Geometry: final body of the model. Coordinates: model frame, mm. Coordinates: 2 decimals unless noted, no trailing zeros. Write each loop counter-clockwise with the first axis right and the second up, starting at its lowest first coordinate (ties: lowest second). Pieces come first, ordered by that corner, then holes. Notation, with made-up numbers: (59.25, 30.5) -> (74.25, 30.5) arc R27 cw to (74.25, 66.5) -> close; hole circle Ø6 at (-8, 82). An arc over 180 degrees is marked (long way). One line per item, written item: value. Start each with the question number.
from build123d import *

# Parameters (mm, degrees)
SKETCH_1_R          = 1.6
EXTRUDE_1_DEPTH     = 3
SKETCH_3_R          = 1.6
CUT_EXTRUDE_1_DEPTH = 92.290744328
FILLET_1_R          = 1
SKETCH_4_W          = 12
SKETCH_4_H          = 3
CUT_EXTRUDE_2_DEPTH = 92.290744328
SKETCH_5_R          = 1
CUT_EXTRUDE_3_DEPTH = 92.290744328
CUT_EXTRUDE_4_DEPTH = 92.290744328
SKETCH_7_R          = 1.6
SKETCH_7_W          = 3
SKETCH_7_H          = 9
EXTRUDE_2_DEPTH     = 3
FILLET_3_R          = 2
SKETCH_8_R          = 1
CUT_EXTRUDE_5_DEPTH = 130.100735862


with BuildPart() as part:
    # 草图1 → 凸台-拉伸1 (new body)
    with BuildSketch(Plane(origin=(0, 0, 0), x_dir=(1, 0, 0), z_dir=(0, 1, 0))):
        Polygon((-90, -15), (-72.5, -15), (-72.5, 0.5), (72.5, 0.5), (72.5, -15), (90, -15), (90, 15), (-90, 15), align=None)
        with Locations(Location((78, -10, 0), (0, 0, 270))):
            Circle(SKETCH_1_R, mode=Mode.SUBTRACT)
        with Locations(Location((-78, -10, 0), (0, 0, 90))):
            Circle(SKETCH_1_R, mode=Mode.SUBTRACT)
        with Locations(Location((-83, 10, 0), (0, 0, 270))):
            Circle(SKETCH_1_R, mode=Mode.SUBTRACT)
        with Locations(Location((83, 10, 0), (0, 0, 90))):
            Circle(SKETCH_1_R, mode=Mode.SUBTRACT)
    extrude(amount=EXTRUDE_1_DEPTH)

    # 草图3 → 切除-拉伸1 (cut, through all)
    with BuildSketch(Plane(origin=(0, 3, 0), x_dir=(1, 0, 0), z_dir=(0, 1, 0))):
        with Locations(Location((87, -4.5, 0), (0, 0, 90))):
            Circle(SKETCH_3_R)
        with Locations(Location((-87, -4.5, 0), (0, 0, 270))):
            Circle(SKETCH_3_R)
    extrude(amount=-CUT_EXTRUDE_1_DEPTH, mode=Mode.SUBTRACT)

    # 圆角1
    fillet_1_edges = [part.edges().sort_by_distance(p)[0] for p in [
        (72.5, 1.5, -0.5),
        (-72.5, 1.5, -0.5),
    ]]
    fillet(fillet_1_edges, radius=FILLET_1_R)

    # 草图4 → 切除-拉伸2 (cut, through all)
    with BuildSketch(Plane.XZ):
        with Locations((60, -7.5)):
            Rectangle(SKETCH_4_W, SKETCH_4_H)
        with Locations((30, -7.5)):
            Rectangle(SKETCH_4_W, SKETCH_4_H)
        with Locations((0, -7.5)):
            Rectangle(SKETCH_4_W, SKETCH_4_H)
        with Locations((-30, -7.5)):
            Rectangle(SKETCH_4_W, SKETCH_4_H)
        with Locations((-60, -7.5)):
            Rectangle(SKETCH_4_W, SKETCH_4_H)
    extrude(amount=-CUT_EXTRUDE_2_DEPTH, mode=Mode.SUBTRACT)

    # 草图5 → 切除-拉伸3 (cut, through all)
    with BuildSketch(Plane.XZ):
        with Locations((65, -9)):
            Circle(SKETCH_5_R)
        with Locations((55, -9)):
            Circle(SKETCH_5_R)
        with Locations((55, -6)):
            Circle(SKETCH_5_R)
        with Locations((65, -6)):
            Circle(SKETCH_5_R)
        with Locations((35, -9)):
            Circle(SKETCH_5_R)
        with Locations((25, -9)):
            Circle(SKETCH_5_R)
        with Locations((25, -6)):
            Circle(SKETCH_5_R)
        with Locations((35, -6)):
            Circle(SKETCH_5_R)
        with Locations((5, -9)):
            Circle(SKETCH_5_R)
        with Locations((-5, -9)):
            Circle(SKETCH_5_R)
        with Locations((-5, -6)):
            Circle(SKETCH_5_R)
        with Locations((5, -6)):
            Circle(SKETCH_5_R)
        with Locations((-25, -9)):
            Circle(SKETCH_5_R)
        with Locations((-35, -9)):
            Circle(SKETCH_5_R)
        with Locations((-35, -6)):
            Circle(SKETCH_5_R)
        with Locations((-25, -6)):
            Circle(SKETCH_5_R)
        with Locations((-55, -9)):
            Circle(SKETCH_5_R)
        with Locations((-65, -9)):
            Circle(SKETCH_5_R)
        with Locations((-65, -6)):
            Circle(SKETCH_5_R)
        with Locations((-55, -6)):
            Circle(SKETCH_5_R)
    extrude(amount=-CUT_EXTRUDE_3_DEPTH, mode=Mode.SUBTRACT)

    # 草图6 → 切除-拉伸4 (cut, through all)
    with BuildSketch(Plane.XZ):
        with BuildLine():
            Line((36.1, -9), (36.1, -6))
            ThreePointArc((36.1, -6), (35.050051841, -4.901139311), (33.904554885, -5.9))
            Line((33.904554885, -5.9), (26.095445115, -5.9))
            ThreePointArc((26.095445115, -5.9), (24.949948159, -4.901139311), (23.9, -6))
            Line((23.9, -6), (23.9, -9))
            ThreePointArc((23.9, -9), (24.949948159, -10.098860689), (26.095445115, -9.1))
            Line((26.095445115, -9.1), (33.904554885, -9.1))
            ThreePointArc((33.904554885, -9.1), (35.050051841, -10.098860689), (36.1, -9))
        make_face()
        with BuildLine():
            Line((66.1, -9), (66.1, -6))
            ThreePointArc((66.1, -6), (65.050051841, -4.901139311), (63.904554885, -5.9))
            Line((63.904554885, -5.9), (56.095445115, -5.9))
            ThreePointArc((56.095445115, -5.9), (54.949948159, -4.901139311), (53.9, -6))
            Line((53.9, -6), (53.9, -9))
            ThreePointArc((53.9, -9), (54.949948159, -10.098860689), (56.095445115, -9.1))
            Line((56.095445115, -9.1), (63.904554885, -9.1))
            ThreePointArc((63.904554885, -9.1), (65.050051841, -10.098860689), (66.1, -9))
        make_face()
        with BuildLine():
            Line((6.1, -9), (6.1, -6))
            ThreePointArc((6.1, -6), (5.050051841, -4.901139311), (3.904554885, -5.9))
            Line((3.904554885, -5.9), (-3.904554885, -5.9))
            ThreePointArc((-3.904554885, -5.9), (-5.050051841, -4.901139311), (-6.1, -6))
            Line((-6.1, -6), (-6.1, -9))
            ThreePointArc((-6.1, -9), (-5.050051841, -10.098860689), (-3.904554885, -9.1))
            Line((-3.904554885, -9.1), (3.904554885, -9.1))
            ThreePointArc((3.904554885, -9.1), (5.050051841, -10.098860689), (6.1, -9))
        make_face()
        with BuildLine():
            Line((-23.9, -9), (-23.9, -6))
            ThreePointArc((-23.9, -6), (-24.949948159, -4.901139311), (-26.095445115, -5.9))
            Line((-26.095445115, -5.9), (-33.904554885, -5.9))
            ThreePointArc((-33.904554885, -5.9), (-35.050051841, -4.901139311), (-36.1, -6))
            Line((-36.1, -6), (-36.1, -9))
            ThreePointArc((-36.1, -9), (-35.050051841, -10.098860689), (-33.904554885, -9.1))
            Line((-33.904554885, -9.1), (-26.095445115, -9.1))
            ThreePointArc((-26.095445115, -9.1), (-24.949948159, -10.098860689), (-23.9, -9))
        make_face()
        with BuildLine():
            Line((-53.9, -9), (-53.9, -6))
            ThreePointArc((-53.9, -6), (-54.949948159, -4.901139311), (-56.095445115, -5.9))
            Line((-56.095445115, -5.9), (-63.904554885, -5.9))
            ThreePointArc((-63.904554885, -5.9), (-65.050051841, -4.901139311), (-66.1, -6))
            Line((-66.1, -6), (-66.1, -9))
            ThreePointArc((-66.1, -9), (-65.050051841, -10.098860689), (-63.904554885, -9.1))
            Line((-63.904554885, -9.1), (-56.095445115, -9.1))
            ThreePointArc((-56.095445115, -9.1), (-54.949948159, -10.098860689), (-53.9, -9))
        make_face()
    extrude(amount=-CUT_EXTRUDE_4_DEPTH, mode=Mode.SUBTRACT)

    # 草图7 → 凸台-拉伸2 (add)
    with BuildSketch(Plane.XZ):
        Polygon((-90, -5.25), (-90, 15), (-93, 15), (-93, 23), (-99, 23), (-99, 10.75), (-127, 10.75), (-127, -5.25), align=None)
        with Locations(Location((-96, 19.75, 0), (0, 0, 270))):
            Circle(SKETCH_7_R, mode=Mode.SUBTRACT)
        with Locations(Location((-106, -2.25, 0), (0, 0, 270))):
            Circle(SKETCH_7_R, mode=Mode.SUBTRACT)
        with Locations((-122.5, 2.75)):
            Rectangle(SKETCH_7_W, SKETCH_7_H, mode=Mode.SUBTRACT)
    extrude(amount=-EXTRUDE_2_DEPTH)

    # 圆角3
    fillet_3_edges = [part.edges().sort_by_distance(p)[0] for p in [
        (90, 1.5, 15),
        (72.5, 1.5, 15),
        (-72.5, 1.5, 15),
        (-90, 1.5, -15),
        (90, 1.5, -15),
        (-93, 1.5, 15),
        (-93, 1.5, 23),
        (-99, 1.5, 23),
        (-99, 1.5, 10.75),
        (-127, 1.5, 10.75),
        (-127, 1.5, -5.25),
        (-90, 1.5, -5.25),
    ]]
    fillet(fillet_3_edges, radius=FILLET_3_R)

    # 草图8 → 切除-拉伸5 (cut, through all)
    with BuildSketch(Plane(origin=(0, 3, 0), x_dir=(1, 0, 0), z_dir=(0, 1, 0))):
        with Locations((-123.5025, 0.882536024)):
            Circle(SKETCH_8_R)
        with Locations((-121.4975, 0.882536024)):
            Circle(SKETCH_8_R)
        with Locations((-121.4975, -6.382536024)):
            Circle(SKETCH_8_R)
        with Locations((-123.5025, -6.382536024)):
            Circle(SKETCH_8_R)
    extrude(amount=-CUT_EXTRUDE_5_DEPTH, mode=Mode.SUBTRACT)


solid = part.part
Q1. Line query: L1, parallel to X at y = 1.35, z = 4.5; L2, parallel to X at y = 1, z = 19.75; L3, parallel to Z at x = 58, y = 1.2. Output: solid intervals per line, ascending. Write a range as from..to.
Q2. First-contact query: P1, Ø1.1, axis at x = -122.5, y = 2, coming from the +Z side; P2, Ø0.9, axis at x = -111, y = 1.5, coming from the -Z side; P3, Ø1.5, axis at y = 2, z = -7, coming from the -X side. Flat tips, straight axial feed; report the tip coordinate or a pass-through.
Q3. Cut plane A-A on y = 2.05. Count the separate pieces of the cut face and the enclosed holes in it, and give its area (3 significant figures).
Q4. Cut plane B-B on x = 45. Output: boundary loops of the cut face in (y, z), and give its area (3 significant figures).
Solution:
1. L1: -127..-124, -121..-88.6, -85.4..-72.5, 72.5..85.4, 88.6..90
1. L2: -99..-97.6, -94.4..-93
1. L3: -15..-9.1, -5.9..-0.5
2. P1: z = 10.75
2. P2: z = -5.25
2. P3: x = -90.27
3. separate pieces: 1
3. enclosed holes: 14
3. area: 3,500 mm²
4. outline: (0, -15) -> (3, -15) -> (3, -0.5) -> (0, -0.5) -> close
4. area: 43.5 mm²
